CAD build for the part. Positions are in the model's coordinates, mm. Coordinates: 2 decimals unless noted, no trailing zeros. Loops run counter-clockwise (first coordinate to the right, second up) from the corner with the lowest first, then second, coordinate; pieces in that order, holes last. Notation, with made-up numbers: (-7, 46.25) -> (16, 46.25) arc R16 cw to (16, 52.25) -> close; hole circle Ø10 at (39.25, 46.25). An arc over 180 degrees is marked (long way). Answer as a JSON object with one key per item and string values. Group by question number.
Autodesk Inventor part; units mm, degrees
ref_plane "YZ Plane" through (0, 0, 0) normal (1, 0, 0) x (0, 1, 0)
ref_plane "XZ Plane" through (0, 0, 0) normal (0, 1, 0) x (-1, 0, 0)
ref_plane "XY Plane" through (0, 0, 0) normal (0, 0, 1) x (1, 0, 0)
sketch "Sketch1" plane through (0, 0, 0) normal (0, 1, 0) x (-1, 0, 0)
  line L0 (59.85, 0) -> (-59.85, 0)
  line L1 (0, -59.85) -> (0, 59.85)
  circle A0 centre (0, 0) radius 42.75
  line L2 (12.5, 12.5) -> (-12.5, 12.5) construction
  line L3 (-12.5, 12.5) -> (-12.5, -12.5) construction
  line L4 (-12.5, -12.5) -> (12.5, -12.5) construction
  line L5 (12.5, -12.5) -> (12.5, 12.5) construction
  circle A1 centre (12.5, 12.5) radius 1.5
  circle A2 centre (-12.5, 12.5) radius 1.5
  circle A3 centre (12.5, -12.5) radius 1.5
  circle A4 centre (-12.5, -12.5) radius 1.5
  circle A5 centre (0, 0) radius 1.5
  dimension "d0" = 85.5
  dimension "d1" = 25
  dimension "d2" = 25
  dimension "d3" = 12.5
  dimension "d4" = 12.5
  dimension "d5" = 3
  dimension "d8" = 25
  dimension "d11" = 25
  dimension "d16" = 3
extrude "Extrusion2" add sketch "Sketch1" along normal blind 1.4 contours A0 L1 A5 L0 | L0 A5 L1 A0 | L1 A5 L0 A0 | A0 L0 A5 L1
sketch "Sketch2" plane through (0, 1.4, 0) normal (0, 1, 0) x (1, 0, 0)
  circle A0 centre (0, 0) radius 1.5
  arc A1 (30, 0) -> (-30, 0) centre (0, 0) ccw
  line L0 (-59.85, 0) -> (59.85, 0)
  line L1 (0, 59.85) -> (0, -59.85)
  arc A2 (42.75, 0) -> (-42.75, 0) centre (0, 0) ccw
  line L2 (-30, 0) -> (-42.75, 0)
  line L3 (30, 0) -> (42.75, 0)
  dimension "d19" = 60
  dimension "d20" = 85.5
extrude "Extrusion3" cut sketch "Sketch2" against normal blind 10 contours A1 L1 A2 L0 | A1 L0 A2 L1
equation "\"d2\" = d1"
equation "\"d3\" = 0.5 * d1"
equation "\"d4\" = 0.5 * d1"
properties part number "PanTilt_Base"
Item 1: Pull direction Z, two halves, no side cores. Call faces 1 (the cylindrical face through (0.66, 0.71, -29.993)), 2 (the cylindrical face through (-11, 0.69, -12.57)), 3 (the flat face through (1, 0, 7)): +Z half, -Z half, draft (parallel to the pull), parting line (faces both ways), or undercut.
Item 2: Band-saw the part on B-B, the plane x = 0. List the corners of the cut face in (y, z), and give its area (4 significant figures).
Item 3: Drill centre lines: L1, parallel to Z at x = -12.5, y = 0.9; L2, parallel to X at y = 0.55, z = -8; L3, parallel to X at y = 1.15, z = 1. Where is each one in solid material? Low to high.
Item 4: Band-saw the part on C-C, the plane z = -12.5. List the corners of the cut face in (x, y), and give its area (3 significant figures).
Item 5: Flat gauge pins, fed straight in: P1, Ø0.7, axis at x = -33.5, y = 1, coming from the -Z side; P2, Ø2.5, axis at x = 12.5, z = 12.5, coming from the +Y side (3 decimals). Where does each tip first touch, or does it go through?
Item 6: Band-saw the part on D-D, the plane x = -12.5. List the corners of the cut face in (y, z), and give its area (3 significant figures).
Item 7: Band-saw the part on A-A, the plane y = 0.4. List the corners of the cut face in (x, z).
Reply:
{
 "1": {"face 1": "-Z half", "face 2": "undercut", "face 3": "draft"},
 "2": {"outline": "(0, -30) -> (1.4, -30) -> (1.4, -1.5) -> (0, -1.5) -> close; (0, 1.5) -> (1.4, 1.5) -> (1.4, 42.75) -> (0, 42.75) -> close", "area": "97.65 mm²"},
 "3": {"L1": "-27.27 to -14, -11 to 11, 14 to 40.88", "L2": "-28.91 to 28.91", "L3": "-42.74 to -1.12, 1.12 to 42.74"},
 "4": {"outline": "(-27.27, 0) -> (-14, 0) -> (-14, 1.4) -> (-27.27, 1.4) -> close; (-11, 0) -> (11, 0) -> (11, 1.4) -> (-11, 1.4) -> close; (14, 0) -> (27.27, 0) -> (27.27, 1.4) -> (14, 1.4) -> close", "area": "68.0 mm²"},
 "5": {"P1": "z = 0", "P2": "through"},
 "6": {"outline": "(0, -27.27) -> (1.4, -27.27) -> (1.4, -14) -> (0, -14) -> close; (0, -11) -> (1.4, -11) -> (1.4, 11) -> (0, 11) -> close; (0, 14) -> (1.4, 14) -> (1.4, 40.88) -> (0, 40.88) -> close", "area": "87.0 mm²"},
 "7": {"outline": "(-42.75, 0) -> (-30, 0) arc R30 ccw to (30, 0) -> (42.75, 0) arc R42.75 ccw to start; hole circle Ø3 at (-12.5, -12.5); hole circle Ø3 at (-12.5, 12.5); hole circle Ø3 at (0, 0); hole circle Ø3 at (12.5, -12.5); hole circle Ø3 at (12.5, 12.5)"}
}
